Geometry check sheet. Reference: the model listing, model coordinates, mm. Face numbers are marked on the shaded views. A direction names the side the tool comes from. Coordinates: 2 decimals unless noted, no trailing zeros. Loops run counter-clockwise (first coordinate to the right, second up) from the corner with the lowest first, then second, coordinate; pieces in that order, holes last.
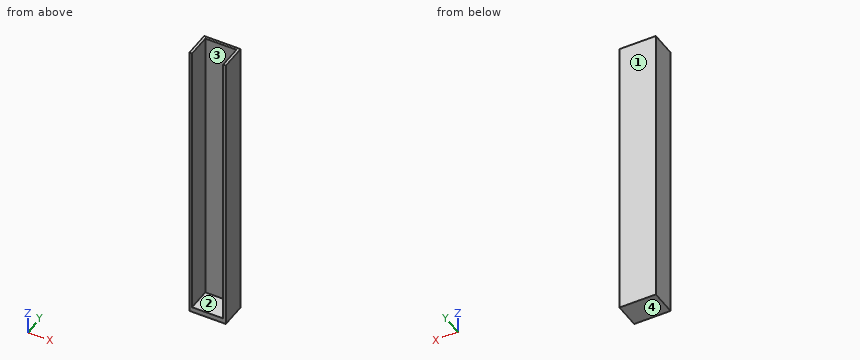
Autodesk Inventor part; units mm, degrees
ref_plane "YZ Plane" through (0, 0, 0) normal (1, 0, 0) x (0, 1, 0)
ref_plane "XZ Plane" through (0, 0, 0) normal (0, 1, 0) x (-1, 0, 0)
ref_plane "XY Plane" through (0, 0, 0) normal (0, 0, 1) x (1, 0, 0)
sketch "Sketch1" plane through (0, 0, 0) normal (0, 0, 1) x (1, 0, 0)
  line L0 (0, 0) -> (28, 0)
  line L1 (28, 0) -> (28, 20)
  line L2 (28, 20) -> (0, 20)
  line L3 (0, 20) -> (0, 0)
  line L4 (2, 18) -> (26, 18)
  line L5 (26, 18) -> (26, 2)
  line L6 (26, 2) -> (2, 2)
  line L7 (2, 2) -> (2, 18)
  line L8 (2, 2) -> (2, 0)
  line L9 (26, 2) -> (26, 0)
  dimension "d0" = 28
  dimension "d1" = 20
  dimension "d2" = 2
extrude "Extrusion1" add sketch "Sketch1" along normal blind 220 contours L3 L2 L1 L0 L9 L5 L4 L7 L8
sketch "Sketch2" plane through (0, 0, 0) normal (0, 0, -1) x (-1, 0, 0)
  line L0 (-28, 20) -> (0, 20)
  line L1 (0, 0) -> (-2, 0)
  line L2 (-28, 20) -> (0, 20)
  line L3 (0, 20) -> (0, 0)
  line L4 (0, 0) -> (-28, 0)
  line L5 (-28, 0) -> (-28, 20)
extrude "Extrusion2" add sketch "Sketch2" along normal blind 4
properties part number "fan_duct"
(1) Access from +Z, -Z, +X, -X, +Y, -Y to the whole of each face (thin tool, end or side, straight path). Record for the marked faces 1 and 2.
Findings:
face 1: +Z, -Z, +X, -X, +Y
face 2: +Z, -Y
(2) Draft check along X on the marked faces 3 and 4. Enter one of: +X half, -X half, draft (parallel to the pull), parting line (faces both ways), or undercut.
Findings:
face 3: undercut
face 4: draft
(3) Gauge pin test, flat ends, axial feed: pin 1 Ø6 at (x, z) = (24, 36.5) entering from -Y; pin 2 Ø5.5 at (x, y) = (16, 7) entering from +Z; pin 3 Ø4 at (x, z) = (14.5, 148.5) entering from -Y. Record the tip position at first contact, or that the pin passes through.
Findings:
pin 1: stops at y = 0
pin 2: stops at z = 0
pin 3: stops at y = 18
(4) Sectioned sample at C-C on x = 8. Record the cut outline in (y, z).
Findings:
outline: (0, -4) - (20, -4) - (20, 220) - (18, 220) - (18, 0) - (0, 0) - close
(5) Scan lines: L1, parallel to X at y = 15.75, z = 28.5; L2, parallel to Z at x = 2.75, y = 13.75; L3, parallel to Y at x = 21, z = 124.5. Record each from-to range of solid material in increasing order.
Findings:
L1: x = 0 to 2, 26 to 28
L2: z = -4 to 0
L3: y = 18 to 20
(6) Sectioned sample at B-B on z = 152.5. Record the cut outline in (x, y).
Findings:
outline: (0, 0) - (2, 0) - (2, 18) - (26, 18) - (26, 0) - (28, 0) - (28, 20) - (0, 20) - close
(7) Sectioned sample at A-A on y = 2. Record the cut outline in (x, z).
Findings:
outline: (0, -4) - (28, -4) - (28, 220) - (26, 220) - (26, 0) - (2, 0) - (2, 220) - (0, 220) - close
